from build123d import *

# Parameters (mm, degrees)
SKETCH1_W             = 100.6348
SKETCH1_H             = 12.7
BOSS_EXTRUDE1_DEPTH   = 3.175
SKETCH2_W             = 3.175
SKETCH2_H             = 12.7
BOSS_EXTRUDE2_DEPTH   = 5.08
SKETCH3_W             = 14.6812
SKETCH3_H             = 12.7
BOSS_EXTRUDE3_DEPTH   = 20.1168
SKETCH4_W             = 8.3312
SKETCH4_H             = 20.1168
CUT_EXTRUDE1_DEPTH    = 20.1168
SKETCH5_W             = 27.1018
SKETCH5_H             = 21.59
BOSS_EXTRUDE4_DEPTH   = 3.175
SKETCH6_W             = 27.1018
SKETCH6_H             = 3.175
BOSS_EXTRUDE5_DEPTH   = 5.08
SKETCH7_W             = 12.7
SKETCH7_H             = 13.335
BOSS_EXTRUDE6_DEPTH   = 3.175
SKETCH8_W             = 12.7
SKETCH8_H             = 3.175
BOSS_EXTRUDE7_DEPTH   = 20.1168
SKETCH9_W             = 12.7
SKETCH9_H             = 3.175
BOSS_EXTRUDE8_DEPTH   = 12.7
SKETCH10_W            = 14.6812
SKETCH10_H            = 3.175
BOSS_EXTRUDE9_DEPTH   = 12.7
F_6_CLEARANCE_HOLE1_D = 3.7973


with BuildPart() as part:
    # Sketch1 → Boss-Extrude1 (new body)
    with BuildSketch(Plane(origin=(0, 0, 0), x_dir=(1, 0, 0), z_dir=(0, 1, 0))):
        Rectangle(SKETCH1_W, SKETCH1_H)
    extrude(amount=BOSS_EXTRUDE1_DEPTH)

    # Sketch2 → Boss-Extrude2 (add)
    with BuildSketch(Plane.XZ):
        with Locations((-48.7299, 0)):
            Rectangle(SKETCH2_W, SKETCH2_H)
        with Locations((48.7299, 0)):
            Rectangle(SKETCH2_W, SKETCH2_H)
    extrude(amount=BOSS_EXTRUDE2_DEPTH)

    # Sketch3 → Boss-Extrude3 (add)
    with BuildSketch(Plane.XZ):
        Rectangle(SKETCH3_W, SKETCH3_H)
    extrude(amount=BOSS_EXTRUDE3_DEPTH)

    # Sketch4 → Cut-Extrude1 (cut)
    with BuildSketch(Plane.XY.offset(6.35)):
        with Locations((0, -6.8834)):
            Rectangle(SKETCH4_W, SKETCH4_H)
    extrude(amount=-CUT_EXTRUDE1_DEPTH, mode=Mode.SUBTRACT)

    # Sketch5 → Boss-Extrude4 (add)
    with BuildSketch(Plane.XZ):
        with Locations((-27.2415, -17.145)):
            Rectangle(SKETCH5_W, SKETCH5_H)
        with Locations((27.2415, -17.145)):
            Rectangle(SKETCH5_W, SKETCH5_H)
    extrude(amount=-BOSS_EXTRUDE4_DEPTH)

    # Sketch6 → Boss-Extrude5 (add)
    with BuildSketch(Plane.XZ):
        with Locations((-27.2415, -26.3525)):
            Rectangle(SKETCH6_W, SKETCH6_H)
        with Locations((27.2415, -26.3525)):
            Rectangle(SKETCH6_W, SKETCH6_H)
    extrude(amount=BOSS_EXTRUDE5_DEPTH)

    # Sketch7 → Boss-Extrude6 (add)
    with BuildSketch(Plane.XZ):
        with Locations((-27.2415, 13.0175)):
            Rectangle(SKETCH7_W, SKETCH7_H)
        with Locations((27.2415, 13.0175)):
            Rectangle(SKETCH7_W, SKETCH7_H)
    extrude(amount=-BOSS_EXTRUDE6_DEPTH)

    # Sketch8 → Boss-Extrude7 (add)
    with BuildSketch(Plane.XZ):
        with Locations((-27.2415, 18.0975)):
            Rectangle(SKETCH8_W, SKETCH8_H)
        with Locations((27.2415, 18.0975)):
            Rectangle(SKETCH8_W, SKETCH8_H)
    extrude(amount=BOSS_EXTRUDE7_DEPTH)

    # Sketch9 → Boss-Extrude8 (add)
    with BuildSketch(Plane.XY.offset(19.685)):
        with Locations((-27.2415, -18.5293)):
            Rectangle(SKETCH9_W, SKETCH9_H)
        with Locations((27.2415, -18.5293)):
            Rectangle(SKETCH9_W, SKETCH9_H)
    extrude(amount=BOSS_EXTRUDE8_DEPTH)

    # Sketch10 → Boss-Extrude9 (add)
    with BuildSketch(Plane(origin=(0, 0, -6.35), x_dir=(-1, 0, 0), z_dir=(0, 0, -1))):
        with Locations((0, -18.5293)):
            Rectangle(SKETCH10_W, SKETCH10_H)
    extrude(amount=BOSS_EXTRUDE9_DEPTH)

    # #6 Clearance Hole1 (through all)
    with Locations(Plane(origin=(0, -16.9418, -12.7), x_dir=(0, 0, 1), z_dir=(0, 1, 0))):
        with Locations((0, 0), (38.735, -27.2415), (38.735, 27.2415)):
            Hole(F_6_CLEARANCE_HOLE1_D / 2)


solid = part.part
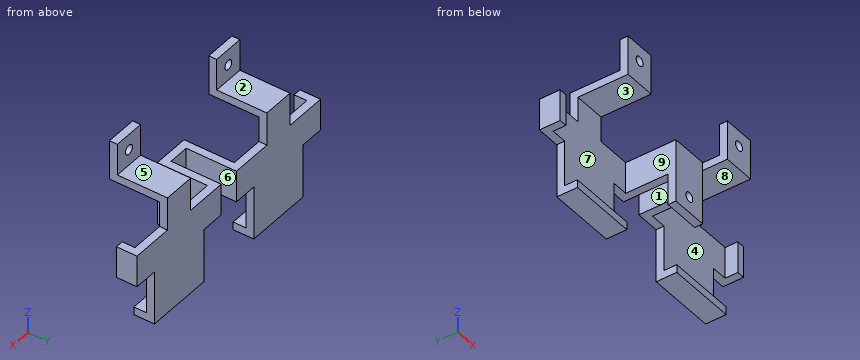
Model file for the job. Use its own axes, mm. Face numbers are marked on the shaded views. A direction names the side the tool comes from. Round coordinates to 2 decimals unless told otherwise and drop trailing zeros. Order: outer loops, then holes, each group sorted by start corner. A loop starts at its lowest first (then second) coordinate and runs counter-clockwise, first axis right, second up.
(1) 3-axis set-ups, long thin cutter, end or side, ignore diameter. For the marked faces 5, 6, 7, 8 and 9: which of +Z, -Z, +X, -X, +Y, -Y reach the whole face in a straight line?
(2) Pin check, flat tips, straight feed: pin 1 (6.5 mm diameter, centred on y = -0.5, z = -18, fed in from -X); pin 2 (8 mm diameter, centred on y = -17.5, z = 14, fed in from +X); pin 3 (10 mm diameter, centred on x = 34, y = -2, fed in from +Z) (3 decimals); pin 4 (5 mm diameter, centred on y = -14, z = -13, fed in from +X). Stop position of each tip, or through.
(3) Band-saw the part on C-C (z = -12.7). List the corners of the cut face in (x, y) (3 decimals), then the cut area to 3 significant figures.
(4) Band-saw the part on A-A (z = 13). List the corners of the cut face in (x, y) (1 decimal).
(5) Drill centre lines: line 1 (X direction, y = -6, z = -0.5); line 2 (Z direction, x = 27, y = -1) (3 decimals); line 3 (X direction, y = -16.75, z = 17.5). Where is each one in solid material? Low to high.
(6) Band-saw the part on B-B (x = 0). List the corners of the cut face in (y, z), then the cut area to 3 significant figures.
(7) Band-saw the part on D-D (y = -11). Give the number of separate pieces and of enclosed holes in the cut face, then the cut area to 3 significant figures.
(8) Pull direction Z, two halves, no side cores. Call the marked faces 1, 2, 3 and 4: released by +Z, released by -Z, zero draft, split by the parting line, or undercut.
Verdict:
1. face 5: +Z, +X, -X, +Y
1. face 6: +Z, -Z, +Y
1. face 7: -Y
1. face 8: +X, -X, -Y
1. face 9: +Z, -Z, -Y
2. pin 1: stops at x = -40.79
2. pin 2: stops at x = 33.59
2. pin 3: stops at z = 19.685
2. pin 4: passes through
3. outline: (-40.792, 0) - (-13.691, 0) - (-13.691, 3.175) - (-40.792, 3.175) - close; (-7.341, -20.117) - (-1.899, -20.117) - (-1.899, -16.942) - (-7.341, -16.942) - close; (1.899, -20.117) - (7.341, -20.117) - (7.341, -16.942) - (1.899, -16.942) - close; (13.691, 0) - (40.792, 0) - (40.792, 3.175) - (13.691, 3.175) - close
3. area: 207 mm2
4. outline: (-33.6, 0) - (-20.9, 0) - (-20.9, 3.2) - (-33.6, 3.2) - close; (20.9, 0) - (33.6, 0) - (33.6, 3.2) - (20.9, 3.2) - close
5. line 1: x = -7.34 to -4.17, 4.17 to 7.34
5. line 2: z = -27.94 to -24.765, 16.51 to 19.685
5. line 3: x = -33.59 to -20.89, 20.89 to 33.59
6. outline: (-20.12, -19.05) - (-16.94, -19.05) - (-16.94, -14.6) - (-20.12, -14.6) - close; (-20.12, -10.8) - (-16.94, -10.8) - (-16.94, 6.35) - (-20.12, 6.35) - close
6. area: 68.6 mm2
7. separate pieces: 4
7. enclosed holes: 0
7. area: 161 mm2
8. face 1: zero draft
8. face 2: released by +Z
8. face 3: undercut
8. face 4: undercut
